Input: dimensioned drawing with shaded views. Units: mm. Origin: part minimum x, y, z. A direction names the side the tool comes from. Give positions to 0.01 mm unless a question says otherwise; leave off trailing zeros. Write each loop counter-clockwise with the first axis right and the second up, starting at its lowest first coordinate (ties: lowest second). Pieces come first, ordered by that corner, then holes. Notation, with made-up numbers: (88, 54) - (142, 54) arc R21 cw to (142, 89) - close; hole circle Ø5 at (34.25, -11.75). An arc over 180 degrees is marked (long way). Answer as a JSON object with one key per item and string values. Group by question number.
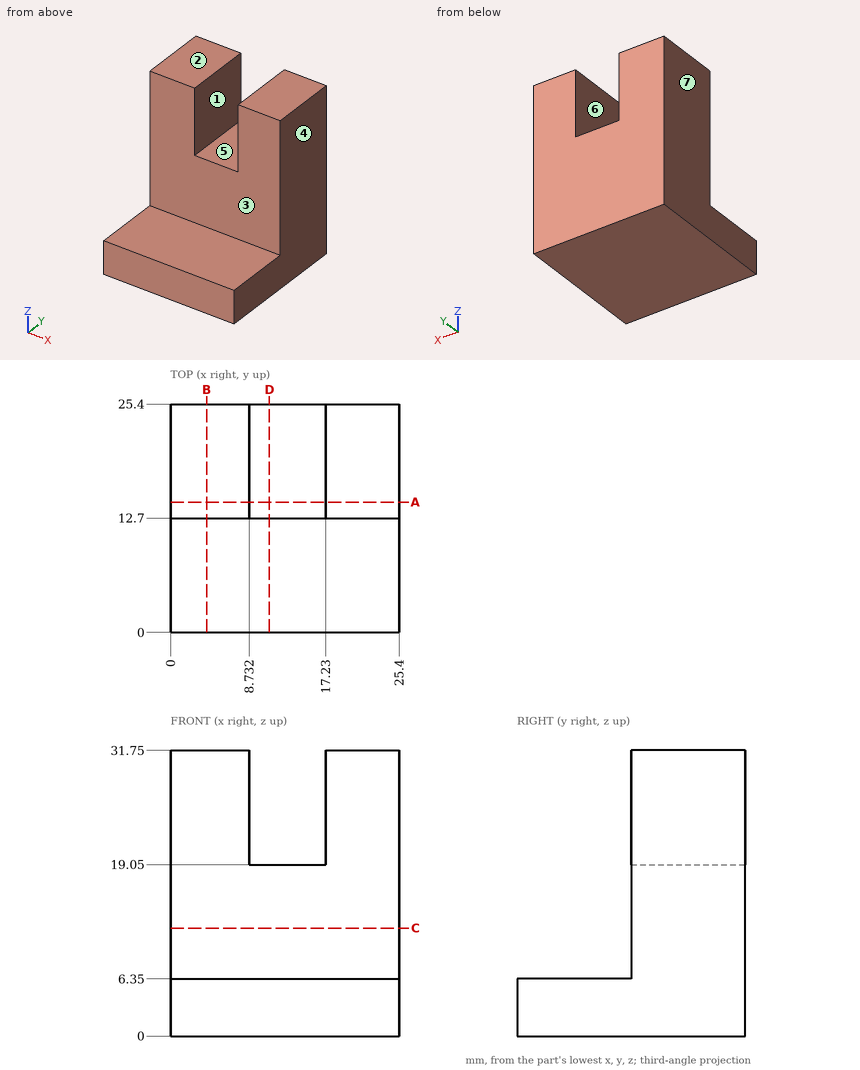
Q1. Section A-A on y = 14.5. Return the cut outline in (x, z).
Q2. First-contact query: pin 1 Ø5 at (y, z) = (14, 10.5) entering from -X; pin 2 Ø4 at (x, y) = (12.5, 5.5) entering from +Z; pin 3 Ø2.5 at (x, y) = (12, 18) entering from +Z. Flat tips, straight axial feed; report the tip coordinate or a pass-through.
Q3. Ray query, probe 1 along X at (y, z) = (20.25, 27); probe 2 along Z at (x, y) = (10.75, 8.5); probe 3 along Y at (x, z) = (14.25, 14). Return the intervals inside material, ascending. Write a range as [from, to].
Q4. Draft query along X for the marked faces 4, 5, 6 and 7. Return one class per face: released by +X, released by -X, zero draft, split by the parting line, or undercut.
Q5. Section D-D on x = 11. Return the cut outline in (y, z).
Q6. Reachability of the marked faces 1, 2 and 3 from +Z, -Z, +X, -X, +Y, -Y: full face, straight path, thin tool, end or side. Return the list, or none.
Q7. Section B-B on x = 4. Return the cut outline in (y, z), then the cut area to 3 significant figures.
Q8. Section C-C on z = 12. Return the cut outline in (x, y), then the cut area to 3 significant figures.
Taken from the geometry:
{
 "1": {"outline": "(0, 0) - (25.4, 0) - (25.4, 31.75) - (17.23, 31.75) - (17.23, 19.05) - (8.73, 19.05) - (8.73, 31.75) - (0, 31.75) - close"},
 "2": {"pin 1": "stops at x = 0", "pin 2": "stops at z = 6.35", "pin 3": "stops at z = 19.05"},
 "3": {"probe 1": "x = [0, 8.73], [17.23, 25.4]", "probe 2": "z = [0, 6.35]", "probe 3": "y = [12.7, 25.4]"},
 "4": {"face 4": "released by +X", "face 5": "undercut", "face 6": "undercut", "face 7": "released by -X"},
 "5": {"outline": "(0, 0) - (25.4, 0) - (25.4, 19.05) - (12.7, 19.05) - (12.7, 6.35) - (0, 6.35) - close"},
 "6": {"face 1": "+Z, +Y, -Y", "face 2": "+Z, +X, -X, +Y, -Y", "face 3": "+Z, +X, -X, -Y"},
 "7": {"outline": "(0, 0) - (25.4, 0) - (25.4, 31.75) - (12.7, 31.75) - (12.7, 6.35) - (0, 6.35) - close", "area": "484 mm²"},
 "8": {"outline": "(0, 12.7) - (25.4, 12.7) - (25.4, 25.4) - (0, 25.4) - close", "area": "323 mm²"}
}
